Verification items for the finished model (mm, model axes). Face numbers are marked on the shaded views. Give positions to 0.01 mm unless a question says otherwise; leave off trailing zeros. Order: outer loops, then holes, each group sorted by start corner. A loop starts at its lowest first (then second) coordinate and runs counter-clockwise, first axis right, second up. Notation, with made-up numbers: (-31, 28) - (-3, 28) arc R22 cw to (-3, 60) - close; hole circle Ø3 at (35, 61.5). An arc over 180 degrees is marked (long way). Answer as a JSON object with one key per item and string values.
```python
from build123d import *

# Parameters (mm, degrees)
SKETCH1_W           = 12
SKETCH1_H           = 90
BOSS_EXTRUDE1_DEPTH = 3
SKETCH2_R           = 3.5
CUT_EXTRUDE1_DEPTH  = 3
SKETCH3_R           = 3
BOSS_EXTRUDE2_DEPTH = 10


with BuildPart() as part:
    # Sketch1 → Boss-Extrude1 (new body)
    with BuildSketch(Plane(origin=(0, 0, 0), x_dir=(0, 0, -1), z_dir=(1, 0, 0))):
        Rectangle(SKETCH1_W, SKETCH1_H)
    extrude(amount=BOSS_EXTRUDE1_DEPTH)

    # Sketch2 → Cut-Extrude1 (cut)
    with BuildSketch(Plane(origin=(3, 0, 0), x_dir=(0, 0, -1), z_dir=(1, 0, 0))):
        with Locations((0, 35)):
            Circle(SKETCH2_R)
    extrude(amount=-CUT_EXTRUDE1_DEPTH, mode=Mode.SUBTRACT)

    # Sketch3 → Boss-Extrude2 (add)
    with BuildSketch(Plane(origin=(3, 0, 0), x_dir=(0, 0, -1), z_dir=(1, 0, 0))):
        with Locations((0, -33)):
            Circle(SKETCH3_R)
    extrude(amount=BOSS_EXTRUDE2_DEPTH)


solid = part.part
```
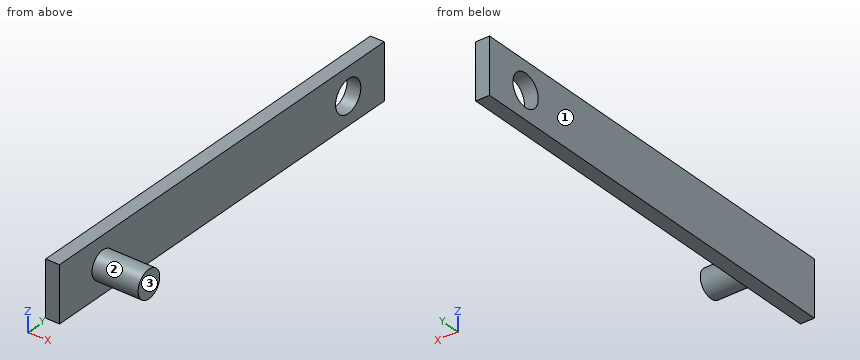
(1) Section check B-B (y = -33). Record the cut outline in (x, z).
Computed values:
{"outline": "(0, -6) - (3, -6) - (3, -3) - (13, -3) - (13, 3) - (3, 3) - (3, 6) - (0, 6) - close"}
(2) Material ranges on line 1 along Y through (x, z) = (1, 0); line 2 along X through (y, z) = (-14.5, 0.5); line 3 along Y through (x, z) = (12, -2), recorded low to high. Write a range as [from, to].
Computed values:
{"line 1": "y = [-45, 31.5], [38.5, 45]", "line 2": "x = [0, 3]", "line 3": "y = [-35.24, -30.76]"}
(3) Section check A-A (z = 0). Record the cut outline in (x, y).
Computed values:
{"outline": "(0, -45) - (3, -45) - (3, -36) - (13, -36) - (13, -30) - (3, -30) - (3, 31.5) - (0, 31.5) - close; (0, 38.5) - (3, 38.5) - (3, 45) - (0, 45) - close"}
(4) Release check for a two-part mould opening along X. For the marked faces 1, 2 and 3 record: pulls with the +X half, pulls with the -X half, needs draft (parallel to the pull), parting line crosses it, or undercut.
Computed values:
{"face 1": "pulls with the -X half", "face 2": "needs draft", "face 3": "pulls with the +X half"}
(5) Section check D-D (x = 5.25). Record the cut outline in (y, z), then the cut area to 3 significant figures.
Computed values:
{"outline": "circle Ø6 at (-33, 0)", "area": "28.3 mm²"}
(6) Section check C-C (y = 35). Record the cut outline in (x, z).
Computed values:
{"outline": "(0, -6) - (3, -6) - (3, -3.5) - (0, -3.5) - close; (0, 3.5) - (3, 3.5) - (3, 6) - (0, 6) - close"}
(7) Gauge pin test, flat ends, axial feed: pin 1 Ø1 at (x, z) = (11.5, -1) entering from -Y; pin 2 Ø6 at (y, z) = (10, 3) entering from +X; pin 3 Ø1.5 at (x, y) = (7, -34) entering from +Z. Record the tip position at first contact, or that the pin passes through.
Computed values:
{"pin 1": "stops at y = -35.96", "pin 2": "stops at x = 3", "pin 3": "stops at z = 2.99"}
